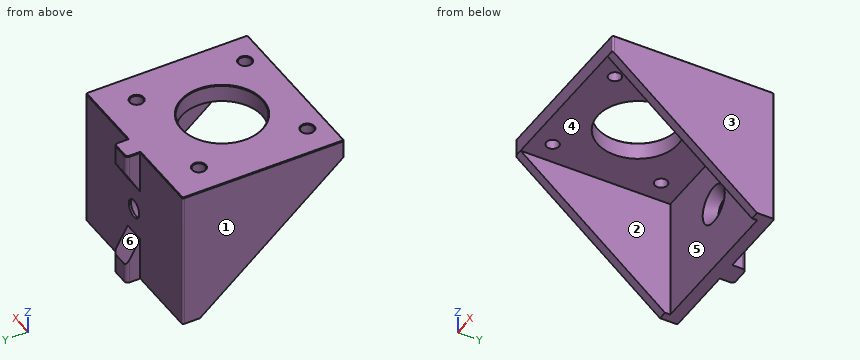
```python
from build123d import *

# Parameters (mm, degrees)
F1_W          = 6.2
F1_H          = 4
F2_DEPTH      = 5
F2_DEPTH_BACK = 35
F3_R          = 1
F5_DEPTH      = 24.151
F5_DEPTH_BACK = 24.151
F6_W          = 43.3
F6_H          = 43.3
F6_R          = 1.8
F6_R_2        = 11.5
F7_DEPTH      = 35.001
F8_DEPTH      = 5.001
F12_R         = 0.5
F13_SIZE      = 0.2


# Not quite as in the source:
# - a feature of the source that left no trace in its solid (it failed there, or was rolled back) is left out


with BuildPart() as f2:
    # F1 (on Top) → F2 (new body, two sides)
    with BuildSketch(Plane.XY) as f2_sk:
        Polygon((-24.15, 25.15), (-24.15, -21.15), (24.15, -21.15), (24.15, 25.15), (3.1, 25.15), (-3.1, 25.15), align=None)
        with Locations((0, 27.15)):
            Rectangle(F1_W, F1_H)
    extrude(amount=F2_DEPTH)
    extrude(f2_sk.sketch, amount=-F2_DEPTH_BACK)

    # F3
    f3_edges = [f2.edges().sort_by_distance(p)[0] for p in [
        (-3.1, 29.15, -15),
        (3.1, 29.15, -15),
    ]]
    fillet(f3_edges, radius=F3_R)

    # F4 (on Right) → F5 (cut, two sides)
    with BuildSketch(Plane.YZ) as f5_sk:
        Polygon((20.15, -35), (-21.15, 0), (-21.15, -35), align=None)
        Polygon((34.9199817246, 9.422104736), (25.15, -7.5), (25.15, -22.5), (34.9199817246, -39.422104736), align=None)
    extrude(amount=-F5_DEPTH, mode=Mode.SUBTRACT)
    extrude(f5_sk.sketch, amount=F5_DEPTH_BACK, mode=Mode.SUBTRACT)

    # F6 (on Top) → F7 (cut, through all)
    with BuildSketch(Plane.XY):
        Rectangle(F6_W, F6_H)
        with Locations((-15.5, -15.5)):
            Circle(F6_R, mode=Mode.SUBTRACT)
        with Locations((15.5, -15.5)):
            Circle(F6_R, mode=Mode.SUBTRACT)
        with Locations((-15.5, 15.5)):
            Circle(F6_R, mode=Mode.SUBTRACT)
        Circle(F6_R_2, mode=Mode.SUBTRACT)
        with Locations((15.5, 15.5)):
            Circle(F6_R, mode=Mode.SUBTRACT)
        with Locations((-15.5, -15.5)):
            Circle(F6_R)
        with Locations((-15.5, 15.5)):
            Circle(F6_R)
        Circle(F6_R_2)
        with Locations((15.5, 15.5)):
            Circle(F6_R)
        with Locations((15.5, -15.5)):
            Circle(F6_R)
    extrude(amount=-F7_DEPTH, mode=Mode.SUBTRACT)

    # F6 (on Top) → F8 (cut, through all)
    with BuildSketch(Plane.XY):
        Circle(F6_R_2)
        with Locations((-15.5, -15.5)):
            Circle(F6_R)
        with Locations((15.5, -15.5)):
            Circle(F6_R)
        with Locations((15.5, 15.5)):
            Circle(F6_R)
        with Locations((-15.5, 15.5)):
            Circle(F6_R)
    extrude(amount=F8_DEPTH, mode=Mode.SUBTRACT)

    # F9 (on Right) → F10 (revolve, cut)
    with BuildSketch(Plane.YZ):
        Polygon((25.15, -17.6), (25.15, -15), (21.65, -15), (21.65, -20.5), (24.55, -17.6), align=None)
    revolve(axis=Axis((0, 23.4, -15), (0, -1, 0)), mode=Mode.SUBTRACT)

    # F12
    f12_edges = [f2.edges().sort_by_distance(p)[0] for p in [
        (24.15, 25.15, -15),
        (-24.15, 25.15, -15),
        (-24.15, -21.15, 2.5),
        (24.15, -21.15, 2.5),
    ]]
    fillet(f12_edges, radius=F12_R)

    # F13
    f13_edges = [f2.edges().sort_by_distance(p)[0] for p in [
        (13.375, 25.15, 5),
        (24.003553, 25.003553, 5),
        (3.1, 26.65, 5),
        (24.15, 2, 5),
        (2.807107, 28.857107, 5),
        (24.003553, -21.003553, 5),
        (0, 29.15, 5),
        (0, -21.15, 5),
        (-2.807107, 28.857107, 5),
        (-24.003553, -21.003553, 5),
        (-3.1, 26.65, 5),
        (-24.15, 2, 5),
        (-13.375, 25.15, 5),
        (-24.003553, 25.003553, 5),
        (-17.3, -15.5, 5),
        (13.7, -15.5, 5),
        (-11.5, 0, 5),
        (-17.3, 15.5, 5),
        (13.7, 15.5, 5),
    ]]
    chamfer(f13_edges, length=F13_SIZE)


solid = f2.part
```
For this review, take the finished solid that the model builds, in its own axes (mm). Face numbers are marked on the shaded views. A direction names the side the tool comes from. Give positions to 0.01 mm unless a question says otherwise; leave off trailing zeros. Loops run counter-clockwise (first coordinate to the right, second up) from the corner with the lowest first, then second, coordinate; pieces in that order, holes last. Notation, with made-up numbers: M 60,24 L 113,24 A25 ccw 113,41 Z; hole C 11.25,-3.5 d4. An arc over 180 degrees is marked long. One line per item, written item: value. Start each with the question number.
Q1. Add section D-D (y = 15.5). Give the boundary of the cut face in (x, z), and give its area (3 significant figures).
Q2. Draft analysis for pull direction X (two halves, no side actions). For the marked faces 3, 4, 5 and 6, state which applies: released by +X, released by -X, zero draft, split by the parting line, or undercut.
Q3. Add section C-C (y = 0). Give the boundary of the cut face in (x, z).
Q4. Clearance check with flat-ended pins moving along their axes: pin 1 Ø3 at (x, y) = (-15.5, -15.5) entering from -Z; pin 2 Ø4 at (x, y) = (15.5, -15.5) entering from -Z; pin 3 Ø0.9 at (y, z) = (27, -30.5) entering from +X; pin 4 Ø3 at (x, z) = (-7.5, -8.5) entering from -Y. State where each tip first meets the part, or that it passes through.
Q5. Machinability: for the marked faces 1 and 2, which of the approach directions +Z, -Z, +X, -X, +Y, -Y give a long, thin tool a straight path to every point of the face, cutting with its end or side? Answer none if there is none.
Q6. Add section A-A (x = 15.5). Give the boundary of the cut face in (y, z), and give its area (3 significant figures).
Q7. Add section B-B (z = -15). Give the boundary of the cut face in (x, y), and give its area (3 significant figures).
Q8. For L1, parallel to X at y = -15.5, z = 2.65; L2, parallel to Y at x = 0, z = 1.6; L3, parallel to X at y = 10, z = -17, list the stretches that pass through material, from the lowest coordinate up.
Reply:
1. outline: M -24.15,-31.06 L -21.65,-31.06 L -21.65,0 L -17.3,0 L -17.3,4.8 L -17.5,5 L -23.95,5 L -24.15,4.8 Z; M -13.7,0 L 13.7,0 L 13.7,4.8 L 13.5,5 L -13.5,5 L -13.7,4.8 Z; M 17.3,0 L 21.65,0 L 21.65,-31.06 L 24.15,-31.06 L 24.15,4.8 L 23.95,5 L 17.5,5 L 17.3,4.8 Z
1. area: 361 mm²
2. face 3: released by +X
2. face 4: undercut
2. face 5: undercut
2. face 6: zero draft
3. outline: M -24.15,-17.92 L -21.65,-17.92 L -21.65,0 L -11.5,0 L -11.5,4.8 L -11.7,5 L -23.95,5 L -24.15,4.8 Z; M 11.5,0 L 21.65,0 L 21.65,-17.92 L 24.15,-17.92 L 24.15,4.8 L 23.95,5 L 11.7,5 L 11.5,4.8 Z
4. pin 1: through
4. pin 2: z = 0
4. pin 3: x = 3.1
4. pin 4: y = 21.65
5. face 1: +Z, -Z, -X, +Y, -Y
5. face 2: -Z, -Y
6. outline: M -21.15,0 L -17.3,0 L -17.3,4.8 L -17.5,5 L -20.95,5 L -21.15,4.8 Z; M -13.7,0 L 13.7,0 L 13.7,4.8 L 13.5,5 L -13.5,5 L -13.7,4.8 Z; M 17.3,0 L 21.65,0 L 21.65,-35 L 25.15,-35 L 25.15,4.8 L 24.95,5 L 17.5,5 L 17.3,4.8 Z
6. area: 318 mm²
7. outline: M -24.15,-3.45 L -21.65,-3.45 L -21.65,21.65 L -5.5,21.65 L -2.6,24.55 L -2.6,25.15 L -23.65,25.15 A0.5 ccw -24.15,24.65 Z; M 2.6,24.55 L 5.5,21.65 L 21.65,21.65 L 21.65,-3.45 L 24.15,-3.45 L 24.15,24.65 A0.5 ccw 23.65,25.15 L 2.6,25.15 Z
7. area: 268 mm²
8. L1: -24.15 to -17.3, -13.7 to 13.7, 17.3 to 24.15
8. L2: -21.15 to -11.5, 11.5 to 29.15
8. L3: -24.15 to -21.65, 21.65 to 24.15
